Check sheet for the modelled part. Datum: model origin and axes. Units: mm. A direction names the side the tool comes from. Round coordinates to 2 decimals unless told otherwise and drop trailing zeros. Write each loop counter-clockwise with the first axis right and the second up, starting at its lowest first coordinate (ties: lowest second). Pieces come first, ordered by that corner, then holes.
Item 1: Material ranges on line 1 (Z direction, x = 9, y = 0.4) (3 decimals); line 2 (Z direction, x = -9, y = 2) (3 decimals); line 3 (X direction, y = 12, z = -7) (3 decimals), recorded low to high.
Item 2: Cross-section at A-A on x = 9. Enter the section's corners in (y, z) (3 decimals).
Item 3: Tool access check on faces 4 (the cylindrical face through (8.6, 1.7, 14.8)), 5 (the flat face through (0, 14, 25.625)), 6 (the cylindrical face through (-8.78, 0.42, 16.44)). Record the directions out of +Z, -Z, +X, -X, +Y, -Y that give a thin tool (end or side, any length) a straight path to the whole face; none if there is none.
Item 4: Go/stop test with flat-tipped pins: pin 1 Ø7.5 at (x, z) = (-8.5, -13.5) entering from +Y; pin 2 Ø5 at (x, y) = (-8.5, 12.5) entering from -Z (3 decimals); pin 3 Ø5 at (x, z) = (-14, 17) entering from -Y; pin 4 Ø5.5 at (x, z) = (-9, -14.875) entering from +Y. Record where each tip stops, or that it passes through.
Item 5: Release check for a two-part mould opening along X. For faces 1 (the flat face through (-18.625, 12, 2)), 2 (the flat face through (0, 13, 28.125)), 3 (the flat face through (-16.125, 14, 1)) record: +X half, -X half, draft (parallel to the pull), parting line (faces both ways), or undercut.
Item 6: Cross-section at D-D on y = 6. Enter the section's corners in (x, z) (3 decimals), plus the area to 3 significant figures.
Item 7: Cross-section at B-B on x = 0. Enter the section's corners in (y, z) (3 decimals), plus the area to 3 significant figures.
Item 8: Cross-section at C-C on z = 13. Enter the section's corners in (x, y) (3 decimals).
from build123d import *

# Parameters (mm, degrees)
SKETCH12_W                      = 32.25
SKETCH12_H                      = 46.25
BOSS_EXTRUDE2_DEPTH             = 2.5
CBORE_FOR_M3_SBHCS1_D           = 3.4
CBORE_FOR_M3_SBHCS1_CBORE_D     = 6.7
CBORE_FOR_M3_SBHCS1_CBORE_DEPTH = 1.65
F_6_0MM_DOWEL_HOLE1_D           = 6.25
SKETCH20_W                      = 46.25
SKETCH20_H                      = 25
BOSS_EXTRUDE3_DEPTH             = 2.5
FILLET1_R                       = 22.7
BOSS_EXTRUDE4_DEPTH             = 2.5
SKETCH23_W                      = 37.25
SKETCH23_H                      = 25
BOSS_EXTRUDE5_DEPTH             = 2.5


with BuildPart() as part:
    # Sketch12 → Boss-Extrude2 (new body)
    with BuildSketch(Plane(origin=(0, 0, 0), x_dir=(1, 0, 0), z_dir=(0, 1, 0))):
        Rectangle(SKETCH12_W, SKETCH12_H)
    extrude(amount=BOSS_EXTRUDE2_DEPTH)

    # CBORE for M3 SBHCS1 (through all)
    with Locations(Plane(origin=(0, 2.5, 0), x_dir=(1, 0, 0), z_dir=(0, 1, 0))):
        with Locations((-9, 14.875), (9, 14.875), (9, -18.125), (-9, -18.125)):
            CounterBoreHole(CBORE_FOR_M3_SBHCS1_D / 2, CBORE_FOR_M3_SBHCS1_CBORE_D / 2, CBORE_FOR_M3_SBHCS1_CBORE_DEPTH)

    # Ø6.0mm Dowel Hole1 (through all)
    with Locations(Plane(origin=(0, 2.5, 0), x_dir=(1, 0, 0), z_dir=(0, 1, 0))):
        with Locations((0, -9.125)):
            Hole(F_6_0MM_DOWEL_HOLE1_D / 2)

    # Sketch20 → Boss-Extrude3 (add)
    with BuildSketch(Plane.ZY.offset(16.125)):
        with Locations((0, 12.5)):
            Rectangle(SKETCH20_W, SKETCH20_H)
    boss_extrude3 = extrude(amount=BOSS_EXTRUDE3_DEPTH)

    # Mirror1: Boss-Extrude3 across plane
    add(boss_extrude3.mirror(Plane.ZY))

    # Fillet1
    fillet1_edges = [part.edges().sort_by_distance(p)[0] for p in [
        (-17.375, 25, -23.125),
    ]]
    fillet(fillet1_edges, radius=FILLET1_R)

    # Sketch22 → Boss-Extrude4 (add)
    with BuildSketch(Plane.XY.offset(23.125)):
        Polygon((-18.625, 0), (18.625, 0), (18.625, 25), (16.125, 25), (16.125, 2.5), (-16.125, 2.5), (-16.125, 25), (-18.625, 25), align=None)
    extrude(amount=BOSS_EXTRUDE4_DEPTH)

    # Sketch23 → Boss-Extrude5 (add)
    with BuildSketch(Plane.XY.offset(25.625)):
        with Locations((0, 12.5)):
            Rectangle(SKETCH23_W, SKETCH23_H)
    extrude(amount=BOSS_EXTRUDE5_DEPTH)


solid = part.part
Response values:
1. line 1: z = -23.125 to -16.575, -13.175 to 16.425, 19.825 to 28.125
1. line 2: z = -23.125 to -18.225, -11.525 to 14.775, 21.475 to 28.125
1. line 3: x = -18.625 to -16.125, 16.125 to 18.625
2. outline: (0, -23.125) - (2.3, -23.125) arc R22.7 ccw to (2.5, -23.124) - (2.5, -18.225) - (0.85, -18.225) - (0.85, -16.575) - (0, -16.575) - close; (0, -13.175) - (0.85, -13.175) - (0.85, -11.525) - (2.5, -11.525) - (2.5, 14.775) - (0.85, 14.775) - (0.85, 16.425) - (0, 16.425) - close; (0, 19.825) - (0.85, 19.825) - (0.85, 21.475) - (2.5, 21.475) - (2.5, 25.625) - (25, 25.625) - (25, 28.125) - (0, 28.125) - close
3. face 4: +Y
3. face 5: -Z, +Y
3. face 6: +Y, -Y
4. pin 1: stops at y = 2.5
4. pin 2: stops at z = 25.625
4. pin 3: stops at y = 0
4. pin 4: stops at y = 0.85
5. face 1: -X half
5. face 2: draft
5. face 3: undercut
6. outline: (-18.625, -22.821) - (-16.125, -22.821) - (-16.125, 25.625) - (16.125, 25.625) - (16.125, -22.821) - (18.625, -22.821) - (18.625, 28.125) - (-18.625, 28.125) - close
6. area: 335 mm2
7. outline: (0, -23.125) - (2.3, -23.125) arc R22.7 ccw to (2.5, -23.124) - (2.5, 6) - (0, 6) - close; (0, 12.25) - (2.5, 12.25) - (2.5, 25.625) - (25, 25.625) - (25, 28.125) - (0, 28.125) - close
7. area: 169 mm2
8. outline: (-18.625, 0) - (18.625, 0) - (18.625, 25) - (16.125, 25) - (16.125, 2.5) - (-16.125, 2.5) - (-16.125, 25) - (-18.625, 25) - close
